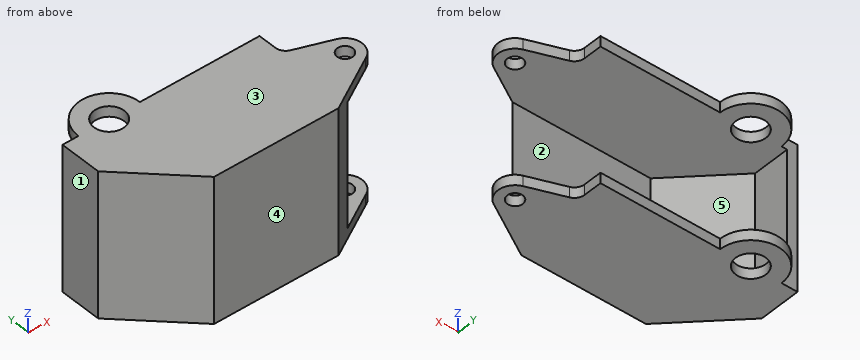
from build123d import *

# Parameters (mm, degrees)
BOSS_EXTRUDE2_DEPTH = 22.58314
SHELL3_T            = -1.6129
SKETCH2_R           = 2.35458
SKETCH2_R_2         = 1.20904
CUT_EXTRUDE1_DEPTH  = 23.58314


with BuildPart() as part:
    # Sketch1 → Boss-Extrude2 (new body)
    with BuildSketch(Plane.XY):
        with BuildLine():
            Line((-17.869818431, 7.881581433), (-20.353938431, 7.881581433))
            Line((-20.353938431, 7.881581433), (-20.353938431, 1.429981433))
            Line((-20.353938431, 1.429981433), (-10.676538431, -8.249958567))
            Line((-10.676538431, -8.249958567), (8.693302541, -8.249958567))
            Line((8.693302541, -8.249958567), (17.046970588, -3.405940625))
            ThreePointArc((17.046970588, -3.405940625), (18.594805131, -0.883615337), (16.848949341, 1.505925245))
            Line((16.848949341, 1.505925245), (11.35487534, 3.505941031))
            ThreePointArc((11.35487534, 3.505941031), (10.585366229, 4.096455714), (10.293701569, 5.021541433))
            Line((10.293701569, 5.021541433), (10.293701569, 7.881581433))
            Line((10.293701569, 7.881581433), (-8.319418431, 7.881581433))
            ThreePointArc((-8.319418431, 7.881581433), (-13.094618431, 12.656781433), (-17.869818431, 7.881581433))
        make_face()
    extrude(amount=BOSS_EXTRUDE2_DEPTH)

    # Shell3
    shell3_openings = [part.faces().sort_by_distance(p)[0] for p in [
        (0.987141569, 7.881581433, 11.29157),
        (10.293701569, 6.451561433, 11.29157),
        (10.704827342, 4.180098473, 11.29157),
        (14.10191234, 2.505933138, 11.29157),
        (17.771382548, -0.916811514, 11.29157),
        (12.870136565, -5.827949596, 11.29157),
        (-19.111878431, 7.881581433, 11.29157),
        (-13.094618431, 10.269181433, 11.29157),
    ]]
    offset(amount=SHELL3_T, openings=shell3_openings, kind=Kind.INTERSECTION)

    # Sketch2 → Cut-Extrude1 (cut, through all)
    with BuildSketch(Plane.XY.offset(22.58314)):
        with Locations((-13.094618431, 7.881581433)):
            Circle(SKETCH2_R)
        with Locations((15.940121569, -0.990638567)):
            Circle(SKETCH2_R_2)
    extrude(amount=-CUT_EXTRUDE1_DEPTH, mode=Mode.SUBTRACT)


solid = part.part
Geometry: final body of the model. Coordinates: model frame, mm. Face numbers are marked on the shaded views. A direction names the side the tool comes from. Round coordinates to 2 decimals unless told otherwise and drop trailing zeros. Order: outer loops, then holes, each group sorted by start corner. A loop starts at its lowest first (then second) coordinate and runs counter-clockwise, first axis right, second up.
Q1. Section A-A, the plane y = 8.5. Output: boundary loops of the cut face in (x, z).
Result sheet:
outline: (-17.83, 0) - (-15.37, 0) - (-15.37, 1.61) - (-17.83, 1.61) - close; (-17.83, 20.97) - (-15.37, 20.97) - (-15.37, 22.58) - (-17.83, 22.58) - close; (-10.82, 0) - (-8.36, 0) - (-8.36, 1.61) - (-10.82, 1.61) - close; (-10.82, 20.97) - (-8.36, 20.97) - (-8.36, 22.58) - (-10.82, 22.58) - close
Q2. Section C-C, the plane z = 12.5. Output: boundary loops of the cut face in (x, y).
Result sheet:
outline: (-20.35, 1.43) - (-10.68, -8.25) - (8.69, -8.25) - (11.47, -6.64) - (-10.01, -6.64) - (-18.74, 2.1) - (-18.74, 7.88) - (-20.35, 7.88) - close
Q3. Section B-B, the plane x = 1.5. Output: boundary loops of the cut face in (y, z), and give its area (3 significant figures).
Result sheet:
outline: (-8.25, 0) - (7.88, 0) - (7.88, 1.61) - (-6.64, 1.61) - (-6.64, 20.97) - (7.88, 20.97) - (7.88, 22.58) - (-8.25, 22.58) - close
area: 83.3 mm2
Q4. Material intervals for probe 1 along Z at (x, y) = (-15, 4.25); probe 2 along X at (y, z) = (2.5, 5); probe 3 along Y at (x, z) = (8, 4.5), sorted ascending.
Result sheet:
probe 1: z = 0 to 1.61, 20.97 to 22.58
probe 2: x = -20.35 to -18.74
probe 3: y = -8.25 to -6.64
Q5. Pin query (flat end, axial travel): pin 1 (1.8 mm diameter, centred on x = -1, z = 22, fed in from +Y); pin 2 (1.7 mm diameter, centred on y = 4.5, z = 13, fed in from +X); pin 3 (1.8 mm diameter, centred on y = 6, z = 22, fed in from +X); pin 4 (1.5 mm diameter, centred on x = -13.5, y = 8, fed in from +Z). Return the tip coordinate at first contact, or that it passes through.
Result sheet:
pin 1: stops at y = 7.88
pin 2: stops at x = -18.74
pin 3: stops at x = 10.29
pin 4: passes through
Q6. Access query for the marked faces 4 and 5. Directions: +Z, -Z, +X, -X, +Y, -Y. A direction counts if a zero-diameter tool reaches every point of the face in a straight line with its end or side. Return the directions, or none.
Result sheet:
face 4: +Z, -Z, +X, -X, -Y
face 5: +X, +Y
Q7. Section D-D, the plane x = 14. Output: boundary loops of the cut face in (y, z).
Result sheet:
outline: (-5.17, 0) - (2.54, 0) - (2.54, 1.61) - (-5.17, 1.61) - close; (-5.17, 20.97) - (2.54, 20.97) - (2.54, 22.58) - (-5.17, 22.58) - close
Q8. Mould query, pull axis Z, two halves, no side actions, for the marked faces 1, 2 and 3. Classes: released by +Z, released by -Z, zero draft, split by the parting line, or undercut.
Result sheet:
face 1: zero draft
face 2: undercut
face 3: released by +Z
